from build123d import *

# Parameters (mm, degrees)
F1_DEPTH = 38.1
F3_DEPTH = 203.2


with BuildPart() as f1:
    # F0 (on Right) → F1 (new body, symmetric)
    with BuildSketch(Plane.YZ):
        with BuildLine():
            ThreePointArc((33.242401, 703.56663), (75.487635, 624.604952), (13.472578, 560.000469))
            Line((13.472578, 560.000469), (-558.8, 457.2))
            Line((-558.8, 457.2), (-914.4, 457.2))
            Line((-914.4, 457.2), (-914.4, 0))
            Line((-914.4, 0), (762, 0))
            Line((762, 0), (762, 1752.6))
            Line((762, 1752.6), (0, 1752.6))
            Line((0, 1752.6), (-914.4, 1752.6))
            Line((-914.4, 1752.6), (-914.4, 1295.4))
            Line((-914.4, 1295.4), (-914.4, 990.6))
            Line((-914.4, 990.6), (-635, 990.6))
            ThreePointArc((-635, 990.6), (-581.118463, 968.281537), (-558.8, 914.4))
            Line((-558.8, 914.4), (-558.8, 779.76663))
            ThreePointArc((-558.8, 779.76663), (-536.481537, 725.885093), (-482.6, 703.56663))
            Line((-482.6, 703.56663), (33.242401, 703.56663))
        make_face()
    extrude(amount=F1_DEPTH, both=True)


with BuildPart() as f3:
    # F2 (on Right) + F1_face (on face) → F3 (new body, symmetric)
    with BuildSketch(Plane.YZ):
        with BuildLine():
            Line((-482.6, 703.56663), (33.242401, 703.56663))
            ThreePointArc((33.242401, 703.56663), (75.487635, 624.604952), (13.472578, 560.000469))
            Line((13.472578, 560.000469), (-558.8, 457.2))
            Line((-558.8, 457.2), (-914.4, 457.2))
            Line((-914.4, 457.2), (-914.4, 0))
            Line((-914.4, 0), (762, 0))
            Line((762, 0), (762, 1752.6))
            Line((762, 1752.6), (-914.4, 1752.6))
            Line((-914.4, 1752.6), (-914.4, 990.6))
            Line((-914.4, 990.6), (-635, 990.6))
            ThreePointArc((-635, 990.6), (-581.118463, 968.281537), (-558.8, 914.4))
            Line((-558.8, 914.4), (-558.8, 779.76663))
            ThreePointArc((-558.8, 779.76663), (-536.481537, 725.885093), (-482.6, 703.56663))
        make_face()
        with BuildLine():
            Line((685.8, 1676.4), (685.8, 76.2))
            Line((685.8, 76.2), (-838.2, 76.2))
            Line((-838.2, 76.2), (-838.2, 381))
            Line((-838.2, 381), (-552.010227, 381))
            Line((-552.010227, 381), (26.945156, 485.000938))
            ThreePointArc((26.945156, 485.000938), (152.026232, 624.333001), (47.627542, 779.76663))
            Line((47.627542, 779.76663), (-482.6, 779.76663))
            Line((-482.6, 779.76663), (-482.6, 914.4))
            ThreePointArc((-482.6, 914.4), (-527.236927, 1022.163073), (-635, 1066.8))
            Line((-635, 1066.8), (-838.2, 1066.8))
            Line((-838.2, 1066.8), (-838.2, 1676.4))
            Line((-838.2, 1676.4), (685.8, 1676.4))
        make_face(mode=Mode.SUBTRACT)
    with BuildSketch(Plane(origin=(38.1, -19.491345, 899.616806), x_dir=(0, 1, 0), z_dir=(1, 0, 0))):
        with BuildLine():
            ThreePointArc((52.733746, -196.050176), (94.97898, -275.011854), (32.963923, -339.616337))
            Line((32.963923, -339.616337), (-539.308655, -442.416806))
            Line((-539.308655, -442.416806), (-894.908655, -442.416806))
            Line((-894.908655, -442.416806), (-894.908655, -899.616806))
            Line((-894.908655, -899.616806), (781.491345, -899.616806))
            Line((781.491345, -899.616806), (781.491345, 852.983194))
            Line((781.491345, 852.983194), (-894.908655, 852.983194))
            Line((-894.908655, 852.983194), (-894.908655, 90.983194))
            Line((-894.908655, 90.983194), (-615.508655, 90.983194))
            ThreePointArc((-615.508655, 90.983194), (-561.627118, 68.664731), (-539.308655, 14.783194))
            Line((-539.308655, 14.783194), (-539.308655, -119.850176))
            ThreePointArc((-539.308655, -119.850176), (-516.990192, -173.731712), (-463.108655, -196.050176))
            Line((-463.108655, -196.050176), (52.733746, -196.050176))
        make_face()
    extrude(amount=F3_DEPTH, both=True)


with BuildPart() as f1_1:
    add(f1.part)

    # F4: union F3
    add(f3.part)


solid = f1_1.part
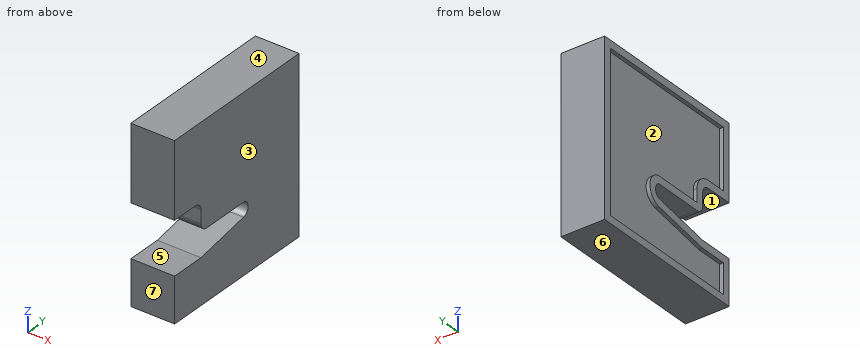
CAD build for the part. Positions are in the model's coordinates, mm. Face numbers are marked on the shaded views. A direction names the side the tool comes from. Give positions to 0.01 mm unless a question says otherwise; leave off trailing zeros. Loops run counter-clockwise (first coordinate to the right, second up) from the corner with the lowest first, then second, coordinate; pieces in that order, holes last. Notation, with made-up numbers: M -32.5,17.25 L 6.5,17.25 A28 ccw 6.5,45.25 Z; hole C 19.25,8 d6. An arc over 180 degrees is marked long. Answer in a Markdown table with one row per item. Add a question column.
Item 1: Band-saw the part on C-C on x = 104. Give the cut face in (y, z), then the cut area to 3 significant figures.
Item 2: Drop flat-ended pins along their axis: P1, Ø5, axis at x = -89, z = 837, coming from the -Y side; P2, Ø12, axis at y = -440.5, z = 1220, coming from the -X side. Give the stop position or say it passes through.
Item 3: Mould opens along Z. For the marked faces 4, 5, 6 and 7 say: +Z half, -Z half, draft (parallel to the pull), parting line (faces both ways), or undercut.
Item 4: Tool access for the marked faces 1, 2 and 3: list every direction of +Z, -Z, +X, -X, +Y, -Y with a clear straight run to the whole face (end or side of a thin tool).
Item 5: Probe probe 1 along Z at (x, y) = (205, -770); probe 2 along X at (y, z) = (576, 417); probe 3 along Z at (x, y) = (-152.5, -422). List the from-to ranges inside material, lowest first.
Item 6: Band-saw the part on A-A on y = -159.5. Give the cut face in (x, z).
Item 7: Band-saw the part on B-B on y = 375.5. Give the cut face in (x, z), then the cut area to 3 significant figures.
Item 8: Band-saw the part on D-D on z = 119.5. Give the cut face in (x, y), then the cut area to 3 significant figures.
Reply:
| question | item | result |
|---|---|---|
| 1 | outline | M -914.4,0 L 762,0 L 762,1752.6 L -914.4,1752.6 L -914.4,990.6 L -635,990.6 A76.2 cw -558.8,914.4 L -558.8,779.77 A76.2 ccw -482.6,703.57 L 33.24,703.57 A76.2 cw 13.47,560 L -558.8,457.2 L -914.4,457.2 Z |
| 1 | area | 2,630,000 mm^2 |
| 2 | P1 | stops at y = -558.8 |
| 2 | P2 | stops at x = -165.1 |
| 3 | face 4 | +Z half |
| 3 | face 5 | undercut |
| 3 | face 6 | -Z half |
| 3 | face 7 | draft |
| 4 | face 1 | +X, -X, -Y |
| 4 | face 2 | -X |
| 4 | face 3 | +Z, -Z, +X, +Y, -Y |
| 5 | probe 1 | z = 0 to 457.2, 990.6 to 1752.6 |
| 5 | probe 2 | x = -165.1 to 241.3 |
| 5 | probe 3 | z = 0 to 481.77, 703.57 to 1752.6 |
| 6 | outline | M -203.2,0 L 241.3,0 L 241.3,528.93 L -203.2,528.93 L -203.2,451.51 L -165.1,451.51 L -165.1,76.2 L -203.2,76.2 Z; M -203.2,703.57 L 241.3,703.57 L 241.3,1752.6 L -203.2,1752.6 L -203.2,1676.4 L -165.1,1676.4 L -165.1,779.77 L -203.2,779.77 Z |
| 7 | outline | M -203.2,0 L 241.3,0 L 241.3,1752.6 L -203.2,1752.6 L -203.2,1676.4 L -165.1,1676.4 L -165.1,76.2 L -203.2,76.2 Z |
| 7 | area | 718,000 mm^2 |
| 8 | outline | M -203.2,-914.4 L 241.3,-914.4 L 241.3,762 L -203.2,762 L -203.2,685.8 L -165.1,685.8 L -165.1,-838.2 L -203.2,-838.2 Z |
| 8 | area | 687,000 mm^2 |
